Geometry: final body of the model. Coordinates: model frame, mm. A direction names the side the tool comes from. Round coordinates to 2 decimals unless told otherwise and drop trailing zeros. Loops run counter-clockwise (first coordinate to the right, second up) from the corner with the lowest first, then second, coordinate; pieces in that order, holes last. Notation, with made-up numbers: M 5.25,-21 L 17.25,-21 A13 ccw 17.25,-12 Z; hole C -36,58 d11. An arc over 180 degrees is marked long. Answer as a JSON object with one key per item and string values.
from build123d import *

# Parameters (mm, degrees)
SKETCH1_W                       = 71.12
SKETCH1_H                       = 71.12
EXTRUDE1_DEPTH                  = 9.525
SKETCH3_R                       = 3.048
CUT_EXTRUDE1_DEPTH              = 10.525
MIRROR3_COPY_1_SKETCH_R         = 3.048
MIRROR3_COPY_1_DEPTH            = 10.525
MIRROR3_COPY_2_SKETCH_R         = 3.048
MIRROR3_COPY_2_DEPTH            = 10.525
SKETCH5_W                       = 10.16
SKETCH5_H                       = 20.32
CUT_EXTRUDE4_DEPTH              = 10.525
SKETCH20_R                      = 13
CUT_EXTRUDE5_DEPTH              = 10.525
CHAMFER1_SIZE                   = 10.16
CHAMFER2_SIZE                   = 10.16
F_6_CLEARANCE_HOLE1_D           = 3.7973
CHAMFER3_SIZE                   = 10.16
SKETCH26_W                      = 50.8
SKETCH26_H                      = 9.525
EXTRUDE2_DEPTH                  = 12.7
F_6_32_TAPPED_HOLE4_D           = 2.7051
F_6_32_TAPPED_HOLE4_DEPTH       = 13.97
F_6_32_TAPPED_HOLE4_CBORE_D     = 3.5052
F_6_32_TAPPED_HOLE4_CBORE_DEPTH = 9.906
F_6_32_TAPPED_HOLE4_TIP         = 0.81269403
F_6_32_TAPPED_HOLE5_D           = 2.7051
F_6_32_TAPPED_HOLE5_DEPTH       = 13.97
F_6_32_TAPPED_HOLE5_TIP         = 0.81269403


with BuildPart() as part:
    # Sketch1 → Extrude1 (new body)
    with BuildSketch(Plane.XY):
        with Locations((-35.56, 35.56)):
            Rectangle(SKETCH1_W, SKETCH1_H)
    extrude(amount=EXTRUDE1_DEPTH)

    # Sketch3 → Cut-Extrude1 (cut, through all)
    with BuildSketch(Plane.XY.offset(9.525)):
        with Locations((-58.908665915, 58.908665915)):
            Circle(SKETCH3_R)
        with Locations((-48.132358569, 48.132358569)):
            Circle(SKETCH3_R)
        Polygon((-58.908665915, 58.908665915), (-56.753404446, 61.063927384), (-45.9770971, 50.287620039), (-50.287620039, 45.9770971), (-61.063927384, 56.753404446), align=None)
    cut_extrude1 = extrude(amount=-CUT_EXTRUDE1_DEPTH, mode=Mode.SUBTRACT)

    # Mirror1: Cut-Extrude1 across plane
    add(cut_extrude1.mirror(Plane.ZX.offset(35.56)), mode=Mode.SUBTRACT)

    # Mirror2: Cut-Extrude1 across plane
    add(cut_extrude1.mirror(Plane(origin=(-35.56, 0, 0), x_dir=(0, 0, 1), z_dir=(1, 0, 0))), mode=Mode.SUBTRACT)

    # Mirror3 copy 1 sketch → Mirror3 copy 1 (cut, through all)
    with BuildSketch(Plane(origin=(-71.12, 71.12, 9.525), x_dir=(-1, 0, 0), z_dir=(0, 0, 1))):
        with Locations((-58.908665915, 58.908665915)):
            Circle(MIRROR3_COPY_1_SKETCH_R)
        with Locations((-48.132358569, 48.132358569)):
            Circle(MIRROR3_COPY_1_SKETCH_R)
        Polygon((-58.908665915, 58.908665915), (-56.753404446, 61.063927384), (-45.9770971, 50.287620039), (-50.287620039, 45.9770971), (-61.063927384, 56.753404446), align=None)
    extrude(amount=-MIRROR3_COPY_1_DEPTH, mode=Mode.SUBTRACT)

    # Mirror3 copy 2 sketch → Mirror3 copy 2 (cut, through all)
    with BuildSketch(Plane(origin=(0, 71.12, 9.525), x_dir=(1, 0, 0), z_dir=(0, 0, 1))):
        with Locations((-58.908665915, -58.908665915)):
            Circle(MIRROR3_COPY_2_SKETCH_R)
        with Locations((-48.132358569, -48.132358569)):
            Circle(MIRROR3_COPY_2_SKETCH_R)
        Polygon((-58.908665915, -58.908665915), (-56.753404446, -61.063927384), (-45.9770971, -50.287620039), (-50.287620039, -45.9770971), (-61.063927384, -56.753404446), align=None)
    extrude(amount=-MIRROR3_COPY_2_DEPTH, mode=Mode.SUBTRACT)

    # Sketch5 → Cut-Extrude4 (cut, through all)
    with BuildSketch(Plane.XY.offset(9.525)):
        with Locations((-35.56, 38.1)):
            Rectangle(SKETCH5_W, SKETCH5_H)
    extrude(amount=-CUT_EXTRUDE4_DEPTH, mode=Mode.SUBTRACT)

    # Sketch20 → Cut-Extrude5 (cut, through all)
    with BuildSketch(Plane.XY.offset(9.525)):
        with Locations((-35.56, -5)):
            Circle(SKETCH20_R)
    extrude(amount=-CUT_EXTRUDE5_DEPTH, mode=Mode.SUBTRACT)

    # Chamfer1
    chamfer1_edges = [part.edges().sort_by_distance(p)[0] for p in [
        (-71.12, 71.12, 4.7625),
    ]]
    chamfer(chamfer1_edges, length=CHAMFER1_SIZE)

    # Chamfer2
    chamfer2_edges = [part.edges().sort_by_distance(p)[0] for p in [
        (0, 71.12, 4.7625),
    ]]
    chamfer(chamfer2_edges, length=CHAMFER2_SIZE)

    # #6 Clearance Hole1 (through all)
    with Locations(Plane(origin=(-45.4025, 31.75, 9.525), x_dir=(1, 0, 0), z_dir=(0, 0, 1))):
        with Locations((0, 0), (-0.0635, 7.619735412)):
            f_6_clearance_hole1 = Hole(F_6_CLEARANCE_HOLE1_D / 2)

    # Mirror11: #6 Clearance Hole1 across plane
    add(f_6_clearance_hole1.mirror(Plane(origin=(-35.56, 0, 0), x_dir=(0, 0, 1), z_dir=(1, 0, 0))), mode=Mode.SUBTRACT)

    # Chamfer3
    chamfer3_edges = [part.edges().sort_by_distance(p)[0] for p in [
        (0, 0, 4.7625),
        (-71.12, 0, 4.7625),
    ]]
    chamfer(chamfer3_edges, length=CHAMFER3_SIZE)

    # Sketch26 → Extrude2 (add)
    with BuildSketch(Plane(origin=(0, 71.12, 0), x_dir=(-1, 0, 0), z_dir=(0, 1, 0))):
        with Locations((35.56, 4.7625)):
            Rectangle(SKETCH26_W, SKETCH26_H)
    extrude(amount=EXTRUDE2_DEPTH)

    # #6-32 Tapped Hole4
    with Locations(Plane(origin=(-53.34, 0, 4.7625), x_dir=(-1, 0, 0), z_dir=(0, -1, 0))):
        with Locations((0, 0), (-35.56, 0)):
            CounterBoreHole(F_6_32_TAPPED_HOLE4_D / 2, F_6_32_TAPPED_HOLE4_CBORE_D / 2, F_6_32_TAPPED_HOLE4_CBORE_DEPTH, depth=F_6_32_TAPPED_HOLE4_DEPTH)
            with Locations((0, 0, -(F_6_32_TAPPED_HOLE4_DEPTH + F_6_32_TAPPED_HOLE4_TIP / 2))):  # 118° drill point
                Cone(0, F_6_32_TAPPED_HOLE4_D / 2, F_6_32_TAPPED_HOLE4_TIP, mode=Mode.SUBTRACT)

    # #6-32 Tapped Hole5
    with Locations(Plane(origin=(-45.466, 83.82, 4.826), x_dir=(1, 0, 0), z_dir=(0, 1, 0))):
        with Locations((0, 0), (19.812, 0)):
            Hole(F_6_32_TAPPED_HOLE5_D / 2, depth=F_6_32_TAPPED_HOLE5_DEPTH)
            with Locations((0, 0, -(F_6_32_TAPPED_HOLE5_DEPTH + F_6_32_TAPPED_HOLE5_TIP / 2))):  # 118° drill point
                Cone(0, F_6_32_TAPPED_HOLE5_D / 2, F_6_32_TAPPED_HOLE5_TIP, mode=Mode.SUBTRACT)


solid = part.part
1) Section query C-C (y = 23). Return the cut outline in (x, z) (3 decimals), and give its area (3 significant figures).
Results:
{"outline": "M -71.12,0 L -52.431,0 L -52.431,9.525 L -71.12,9.525 Z; M -45.084,0 L -26.036,0 L -26.036,9.525 L -45.084,9.525 Z; M -18.689,0 L 0,0 L 0,9.525 L -18.689,9.525 Z", "area": "537 mm2"}
2) Reachability of faces 4 (the cylindrical face through (-46.756, 76.737, 4.42)), 5 (the flat face through (-55.6, 19.83, 4.83)), 6 (the cylindrical face through (-52.05, 11.51, 4.36)) from +Z, -Z, +X, -X, +Y, -Y: full face, straight path, thin tool, end or side. Return the list, or none.
Results:
{"face 4": "+Y", "face 5": "+Z, -Z", "face 6": "-Y"}
3) Ray query, line 1 (X direction, y = 76, z = 5); line 2 (X direction, y = 41, z = 7.25); line 3 (X direction, y = 10, z = 6). Return the intervals inside material, ascending.
Results:
{"line 1": "-60.96 to -46.81, -44.12 to -27, -24.31 to -10.16", "line 2": "-71.12 to -46.44, -44.49 to -40.64, -30.48 to -26.63, -24.68 to 0", "line 3": "-70.96 to -61.01, -56.81 to -53.89, -52.79 to -18.33, -17.23 to -14.31, -10.11 to -0.16"}
4) Section query B-B (x = -48.5). Return the cut outline in (y, z) (3 decimals).
Results:
{"outline": "M 0,0 L 18.309,0 L 18.309,9.525 L 0,9.525 Z; M 26.013,0 L 45.107,0 L 45.107,9.525 L 26.013,9.525 Z; M 52.811,0 L 83.82,0 L 83.82,9.525 L 52.811,9.525 Z"}
5) Section query D-D (x = -31.5). Return the cut outline in (y, z) (3 decimals).
Results:
{"outline": "M 7.35,0 L 27.94,0 L 27.94,9.525 L 7.35,9.525 Z; M 48.26,0 L 83.82,0 L 83.82,9.525 L 48.26,9.525 Z"}
6) Pin query (flat end, axial travel): P1, Ø2.5, axis at x = -25.72, y = 31.75, coming from the +Z side; P2, Ø4.5, axis at x = -45.466, z = 4.826, coming from the +Y side; P3, Ø1.1, axis at x = -17, z = 4, coming from the -Y side; P4, Ø2, axis at x = -25.654, z = 4.826, coming from the +Y side. Return the tip coordinate at first contact, or that it passes through.
Results:
{"P1": "through", "P2": "y = 83.82", "P3": "y = 9.91", "P4": "y = 69.64"}
7) Section query A-A (y = 31.75). Return the cut outline in (x, z) (3 decimals).
Results:
{"outline": "M -71.12,0 L -47.301,0 L -47.301,9.525 L -71.12,9.525 Z; M -43.504,0 L -40.64,0 L -40.64,9.525 L -43.504,9.525 Z; M -30.48,0 L -27.616,0 L -27.616,9.525 L -30.48,9.525 Z; M -23.819,0 L 0,0 L 0,9.525 L -23.819,9.525 Z"}
8) Pull-direction query (Z, two-part tool) for faces 1 (the flat face through (-35, 51, 9.525)), 2 (the cylindrical face through (-26.944, 76.737, 4.42)), 3 (the flat face through (-60.96, 77, 5)); classes: +Z half, -Z half, draft (parallel to the pull), parting line (faces both ways), or undercut.
Results:
{"face 1": "+Z half", "face 2": "undercut", "face 3": "draft"}
